The listing builds one solid part. Answer for the finished solid, in the listing's coordinates (mm). Coordinates: 2 decimals unless noted, no trailing zeros. Loops run counter-clockwise (first coordinate to the right, second up) from the corner with the lowest first, then second, coordinate; pieces in that order, holes last. Notation, with made-up numbers: (57, -23) - (113, -23) arc R28 cw to (113, -4) - close; hole circle Ø1 at (74, 22). An arc over 180 degrees is marked (long way). One line per question, with ' | ' between items.
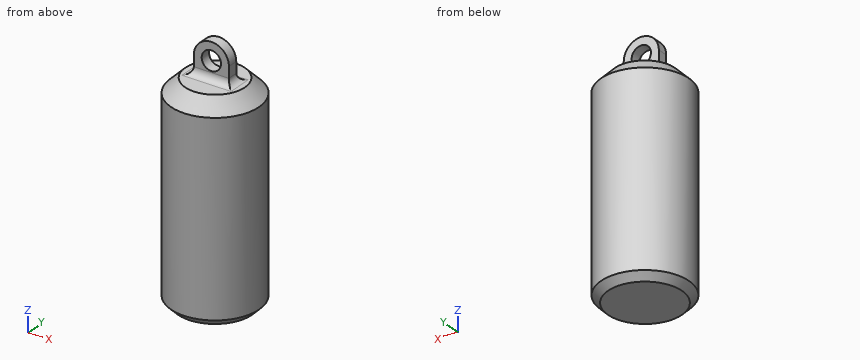
from build123d import *

# Parameters (mm, degrees)
SKETCH4_R           = 2.75
BOSS_EXTRUDE1_DEPTH = 1.5
BOSS_EXTRUDE2_START = 45
SKETCH5_R           = 12.5
BOSS_EXTRUDE2_DEPTH = 45
CHAMFER1_SIZE       = 4
FILLET1_R           = 2
CHAMFER2_SIZE       = 2


with BuildPart() as part:
    # Sketch3 → Revolve2 (revolve)
    with BuildSketch(Plane(origin=(0, 0, 0), x_dir=(0, 0, -1), z_dir=(1, 0, 0)), mode=Mode.PRIVATE) as revolve2_sk:
        Polygon((-4.082352568, 12.5), (4.082352568, 12.5), (4.082352568, 0), (-10.590979782, 0), (-10.590979782, 12.5), align=None)
    revolve(revolve2_sk.sketch.rotate(Axis((0, 0, 16.393474527), (0, 0, -1)), 90), axis=Axis((0, 0, 16.393474527), (0, 0, -1)))

    # Sketch4 → Boss-Extrude1 (add, symmetric)
    with BuildSketch(Plane(origin=(0, 0, 0), x_dir=(1, 0, 0), z_dir=(0, 1, 0))):
        with BuildLine():
            Line((-5, -15.723809824), (-5, -10.590979782))
            Line((-5, -10.590979782), (5, -10.590979782))
            Line((5, -10.590979782), (5, -15.723809824))
            ThreePointArc((5, -15.723809824), (0, -20.723809824), (-5, -15.723809824))
        make_face()
        with Locations(Location((0, -15.723809824, 0), (0, 0, 270))):
            Circle(SKETCH4_R, mode=Mode.SUBTRACT)
    extrude(amount=BOSS_EXTRUDE1_DEPTH, both=True)

    # Sketch5 → Boss-Extrude2 (add)
    with BuildSketch(Plane(origin=(0, 0, -4.082352568), x_dir=(-1, 0, 0), z_dir=(0, 0, -1)).offset(BOSS_EXTRUDE2_START)):
        with Locations(Location((0, 0, 0), (0, 0, 180))):
            Circle(SKETCH5_R)
    extrude(amount=-BOSS_EXTRUDE2_DEPTH)

    # Chamfer1
    chamfer1_edges = [part.edges().sort_by_distance(p)[0] for p in [
        (-12.5, 0, 10.590979782),
    ]]
    chamfer(chamfer1_edges, length=CHAMFER1_SIZE)

    # Fillet1
    fillet1_edges = [part.edges().sort_by_distance(p)[0] for p in [
        (0, 1.5, 10.590979782),
        (0, -1.5, 10.590979782),
        (5, 0, 10.590979782),
        (-5, 0, 10.590979782),
    ]]
    fillet(fillet1_edges, radius=FILLET1_R)

    # Chamfer2
    chamfer2_edges = [part.edges().sort_by_distance(p)[0] for p in [
        (-12.5, 0, -49.082352568),
    ]]
    chamfer(chamfer2_edges, length=CHAMFER2_SIZE)


solid = part.part
Item 1: Find the intervals of material crossed by line 1 (Z direction, x = -2.5, y = 5.25); line 2 (X direction, y = -0.25, z = -26); line 3 (X direction, y = 5.5, z = -4.5), in increasing order. Write a range as [from, to].
Taken from the geometry:
line 1: z = [-49.08, 10.59] | line 2: x = [-12.5, 12.5] | line 3: x = [-11.22, 11.22]
Item 2: Each of these flat-tipped pins is pushed along its axis until it touches: pin 1 Ø10 at (y, z) = (6, -15.5) entering from +X; pin 2 Ø1 at (y, z) = (4.5, -22.5) entering from -X; pin 3 Ø1 at (x, y) = (6, 9.5) entering from -Z. Where does it stop, or does it pass through?
Taken from the geometry:
pin 1: stops at x = 12.46 | pin 2: stops at x = -11.84 | pin 3: stops at z = -48.85
Item 3: Find section B-B, the plane z = -2. Write down the section's boundary in (x, y), plus the area to 3 significant figures.
Taken from the geometry:
outline: circle Ø25 at (0, 0) | area: 491 mm2
Item 4: Find section A-A, the plane y = 0. Write down the section's boundary in (x, z).
Taken from the geometry:
outline: (-12.5, -47.08) - (-10.5, -49.08) - (10.5, -49.08) - (12.5, -47.08) - (12.5, 6.59) - (8.5, 10.59) - (7, 10.59) arc R2 cw to (5, 12.59) - (5, 15.72) arc R5 ccw to (-5, 15.72) - (-5, 12.59) arc R2 cw to (-7, 10.59) - (-8.5, 10.59) - (-12.5, 6.59) - close; hole circle Ø5.5 at (0, 15.72)
Item 5: Find section C-C, the plane z = 8. Write down the section's boundary in (x, y), plus the area to 3 significant figures.
Taken from the geometry:
outline: circle Ø22.18 at (0, 0) | area: 386 mm2
